```python
from build123d import *

# Parameters (mm, degrees)
SKETCH_R        = 25
PAD_DEPTH       = 25
PAD_TAPER       = 15
SKETCH001_R     = 17.5
POCKET_DEPTH    = 20
POCKET_TAPER    = 15
SKETCH002_R     = 10
PAD001_DEPTH    = 20
PAD001_TAPER    = 18
SKETCH003_R     = 1.5
POCKET001_DEPTH = 17


with BuildPart() as part:
    # Sketch → Pad (new body)
    with BuildSketch(Plane.XY):
        Circle(SKETCH_R)
    extrude(amount=PAD_DEPTH, taper=PAD_TAPER)

    # Sketch001 (on Face2 of Pad) → Pocket (cut)
    with BuildSketch(Plane(origin=(0, 0, 0), x_dir=(1, 0, 0), z_dir=(0, 0, -1))):
        Circle(SKETCH001_R)
    extrude(amount=-POCKET_DEPTH, taper=POCKET_TAPER, mode=Mode.SUBTRACT)

    # Sketch002 (on Face5 of Pocket) → Pad001 (join)
    with BuildSketch(Plane(origin=(0, 0, 20), x_dir=(1, 0, 0), z_dir=(0, 0, -1))):
        Circle(SKETCH002_R)
    extrude(amount=PAD001_DEPTH, taper=PAD001_TAPER)

    # Sketch003 (on Face7 of Pad001) → Pocket001 (cut)
    with BuildSketch(Plane(origin=(0, 0, 0), x_dir=(1, 0, 0), z_dir=(0, 0, -1))):
        Circle(SKETCH003_R)
    extrude(amount=-POCKET001_DEPTH, mode=Mode.SUBTRACT)


solid = part.part
```
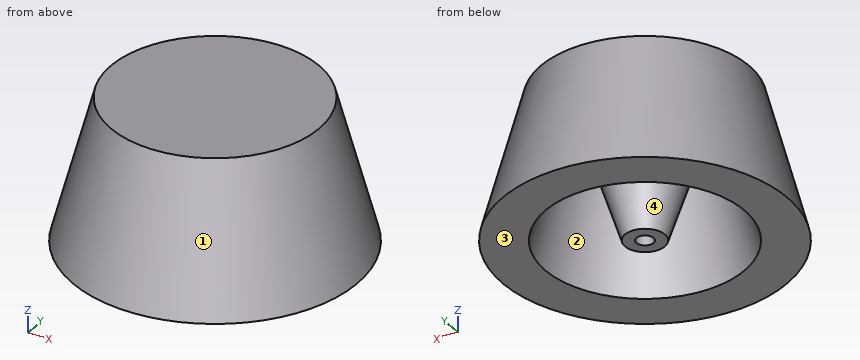
The model under review builds one solid part; all positions refer to its coordinate system, in mm. Face numbers are marked on the shaded views. Give positions to 0.01 mm unless a question says otherwise; leave off trailing zeros. Write each loop counter-clockwise with the first axis right and the second up, starting at its lowest first coordinate (ties: lowest second). Pieces come first, ordered by that corner, then holes. Notation, with made-up numbers: M -12.75,-1 L 43.25,-1 A15 ccw 43.25,14 Z; hole C 0,-12 d4. An arc over 180 degrees is marked long. Write item = value, one per line. Start each with the question number.
Q1. For line 1 (X direction, y = 3.5, z = 14.25); line 2 (Y direction, x = 0, z = 13.5); line 3 (Y direction, x = -4, z = 4.5), list the stretches that pass through material, from the lowest coordinate up.
Q2. Mouldability with a two-part tool opening along Y and no side actions: class the marked faces 1, 2, 3 and 4 as released by +Y, released by -Y, zero draft, split by the parting line, or undercut.
Q3. Clearance check with flat-ended pins moving along their axes: pin 1 (4 mm diameter, centred on y = 1, z = 21, fed in from +X); pin 2 (4 mm diameter, centred on y = 17, z = 17.5, fed in from +X); pin 3 (8 mm diameter, centred on y = -3, z = 18, fed in from -X). State where each tip first meets the part, or that it passes through.
Q4. We need section D-D (z = 22.5). State the section outline as (x, y) points, plus the area to 3 significant figures.
Q5. We need section A-A (x = 0). State the section outline as (y, z) points.
Q6. We need section B-B (z = 13.25). State the section outline as (x, y) points, plus the area to 3 significant figures.
Q7. We need section C-C (z = 16). State the section outline as (x, y) points.
Result set:
q1.line_1 = -20.89 to -13.23, -7.34 to 7.34, 13.23 to 20.89
q1.line_2 = -21.38 to -13.88, -7.89 to -1.5, 1.5 to 7.89, 13.88 to 21.38
q1.line_3 = -23.46 to -15.8, -2.94 to 2.94, 15.8 to 23.46
q2.face_1 = split by the parting line
q2.face_2 = undercut
q2.face_3 = zero draft
q2.face_4 = undercut
q3.pin_1 = 19.89
q3.pin_2 = 13.83
q3.pin_3 = -21.12
q4.outline = C 0,0 d37.94
q4.area = 1,130 mm2
q5.outline = M -25,0 L -17.5,0 L -12.14,20 L -10,20 L -3.5,0 L -1.5,0 L -1.5,17 L 1.5,17 L 1.5,0 L 3.5,0 L 10,20 L 12.14,20 L 17.5,0 L 25,0 L 18.3,25 L -18.3,25 Z
q6.outline = C 0,0 d42.9; C 0,0 d15.61; hole C 0,0 d27.9; hole C 0,0 d3
q6.area = 1,020 mm2
q7.outline = C 0,0 d41.43; C 0,0 d17.4; hole C 0,0 d26.43; hole C 0,0 d3
